For this review, take the finished solid that the model builds, in its own axes (mm). A direction names the side the tool comes from. Coordinates: 2 decimals unless noted, no trailing zeros. Loops run counter-clockwise (first coordinate to the right, second up) from the corner with the lowest first, then second, coordinate; pieces in that order, holes last. Notation, with made-up numbers: M 36,32.5 L 42,32.5 A19 ccw 42,40.5 Z; hole C -20,85.5 d10. An arc over 180 degrees is marked long. Use one line per item in the form item = value.
```python
from build123d import *

# Parameters (mm, degrees)
SKETCH1_W                = 42.3
SKETCH1_H                = 42.3
BOSS_EXTRUDE1_DEPTH      = 50
SKETCH2_R                = 11
BOSS_EXTRUDE2_DEPTH      = 2
SKETCH3_R                = 1.75
CUT_EXTRUDE1_DEPTH       = 51
CUT_EXTRUDE2_DEPTH       = 51
SKETCH5_R                = 2.5
CUT_EXTRUDE3_DEPTH       = 53
SKETCH6_R                = 2.5
BOSS_EXTRUDE3_DEPTH      = 22
BOSS_EXTRUDE3_DEPTH_BACK = 52
SKETCH7_R                = 5
SKETCH7_R_2              = 2.5
CUT_EXTRUDE4_DEPTH       = 5
CUT_EXTRUDE5_DEPTH       = 20
SKETCH9_OUTSIDE_W        = 63.332
SKETCH9_OUTSIDE_H        = 63.332
SKETCH9_OUTSIDE_R        = 2.5
CUT_EXTRUDE6_DEPTH       = 75


with BuildPart() as part:
    # Sketch1 → Boss-Extrude1 (new body)
    with BuildSketch(Plane.XY):
        Rectangle(SKETCH1_W, SKETCH1_H)
    extrude(amount=BOSS_EXTRUDE1_DEPTH)

    # Sketch2 → Boss-Extrude2 (add)
    with BuildSketch(Plane.XY.offset(50)):
        Circle(SKETCH2_R)
    extrude(amount=BOSS_EXTRUDE2_DEPTH)

    # Sketch3 → Cut-Extrude1 (cut, through all)
    with BuildSketch(Plane.XY.offset(50)):
        with Locations((-16.55, 16.55)):
            Circle(SKETCH3_R)
        with Locations((16.55, 16.55)):
            Circle(SKETCH3_R)
        with Locations((16.55, -16.55)):
            Circle(SKETCH3_R)
        with Locations((-16.55, -16.55)):
            Circle(SKETCH3_R)
    extrude(amount=-CUT_EXTRUDE1_DEPTH, mode=Mode.SUBTRACT)

    # Sketch4 → Cut-Extrude2 (cut, through all)
    with BuildSketch(Plane.XY.offset(50)):
        Polygon((-21.15, 17.897308807), (-21.15, 21.15), (-17.897308807, 21.15), align=None)
        Polygon((17.897308807, 21.15), (21.15, 21.15), (21.15, 17.897308807), align=None)
        Polygon((21.15, -17.897308807), (21.15, -21.15), (17.897308807, -21.15), align=None)
        Polygon((-17.897308807, -21.15), (-21.15, -21.15), (-21.15, -17.897308807), align=None)
    extrude(amount=-CUT_EXTRUDE2_DEPTH, mode=Mode.SUBTRACT)

    # Sketch5 → Cut-Extrude3 (cut, through all)
    with BuildSketch(Plane.XY.offset(52)):
        Circle(SKETCH5_R)
    extrude(amount=-CUT_EXTRUDE3_DEPTH, mode=Mode.SUBTRACT)

    # Sketch6 → Boss-Extrude3 (add, two sides)
    with BuildSketch(Plane.XY.offset(52)) as boss_extrude3_sk:
        Circle(SKETCH6_R)
    extrude(amount=BOSS_EXTRUDE3_DEPTH)
    extrude(boss_extrude3_sk.sketch, amount=-BOSS_EXTRUDE3_DEPTH_BACK)

    # Sketch7 → Cut-Extrude4 (cut)
    with BuildSketch(Plane(origin=(0, 0, 0), x_dir=(-1, 0, 0), z_dir=(0, 0, -1))):
        Circle(SKETCH7_R)
        Circle(SKETCH7_R_2, mode=Mode.SUBTRACT)
    extrude(amount=-CUT_EXTRUDE4_DEPTH, mode=Mode.SUBTRACT)

    # Sketch8 → Cut-Extrude5 (cut)
    with BuildSketch(Plane.XY.offset(74)):
        with BuildLine():
            Line((2.5, 0), (0, 2.5))
            ThreePointArc((0, 2.5), (1.767766953, 1.767766953), (2.5, 0))
        make_face()
    extrude(amount=-CUT_EXTRUDE5_DEPTH, mode=Mode.SUBTRACT)

    # Sketch9 outside → Cut-Extrude6 (cut, through all)
    with BuildSketch(Plane.XY.offset(74)):
        Rectangle(SKETCH9_OUTSIDE_W, SKETCH9_OUTSIDE_H)
        Circle(SKETCH9_OUTSIDE_R, mode=Mode.SUBTRACT)
    extrude(amount=-CUT_EXTRUDE6_DEPTH, mode=Mode.SUBTRACT)


solid = part.part
```
1. Wall thickness on line 1 along Y through (x, z) = (0.15, 13); line 2 along X through (y, z) = (0.25, 37); line 3 along Z through (x, y) = (1.8, 1.5): over which ranges is each line inside the solid? List them lowest first. Write a range as from..to.
Computed values:
line_1 = -2.5..2.5
line_2 = -2.49..2.49
line_3 = 0..54
2. Tool access review of faces 1 (the face through (0, 0, 0)), 2 (the face through (1.3, 1.2, 64.1)): name each direction out of +Z, -Z, +X, -X, +Y, -Y from which nothing blocks a thin tool from reaching the whole face with its end or side.
Computed values:
face_1 = -Z, +X, -X, +Y, -Y
face_2 = +Z, +X, +Y
3. Consider section C-C on y = 1.55. Write out the cut boundary in (x, z).
Computed values:
outline = M -1.96,0 L 1.96,0 L 1.96,54 L 0.95,54 L 0.95,74 L -1.96,74 Z
4. Consider section D-D on z = 58.5. Write out the cut boundary in (x, y).
Computed values:
outline = M 0,2.5 A2.5 ccw long 2.5,0 Z
5. Consider section B-B on z = 17.5. Write out the cut boundary in (x, y), plus the area to 3 significant figures.
Computed values:
outline = C 0,0 d5
area = 19.6 mm2
6. Consider section A-A on x = 0.7. Write out the cut boundary in (y, z), plus the area to 3 significant figures.
Computed values:
outline = M -2.4,0 L 2.4,0 L 2.4,54 L 1.8,54 L 1.8,74 L -2.4,74 Z
area = 343 mm2
